The drawing under review shows one solid part. Ordinate dimensions are in mm from its lowest x, y, z. Round coordinates to 2 decimals unless told otherwise and drop trailing zeros. Write each loop counter-clockwise with the first axis right and the second up, starting at its lowest first coordinate (ties: lowest second). Pieces come first, ordered by that corner, then holes. Notation, with made-up numbers: M -6,52 L 46,52 A32 ccw 46,84 Z; hole C -6,2 d8. An arc over 180 degrees is marked long. One line per item, written item: value. Start each with the question number.
1) Take a section at C-C, the plane y = 4.5. Write out the cut boundary in (x, z) (3 decimals).
2) Wall thickness on probe 1 along X at (y, z) = (3, 62.5) (3 decimals); probe 2 along Z at (x, y) = (109.5, 2) (3 decimals); probe 3 along Z at (x, y) = (108.5, 6.25) (3 decimals): over which ranges is each line inside the solid? List them lowest first.
3) For P1, Ø4, axis at x = 117.475, z = 122.809, coming from the +Y side (3 decimals); P2, Ø3, axis at x = 3.175, z = 13.589, coming from the -Y side, all flat-tipped, find the tip position at first contact; note any pin that passes through.
4) Take a section at B-B, the plane z = 67. Write out the cut boundary in (x, y) (3 decimals).
5) Take a section at A-A, the plane x = 191. Write out the cut boundary in (y, z) (3 decimals), and give its area (3 significant figures).
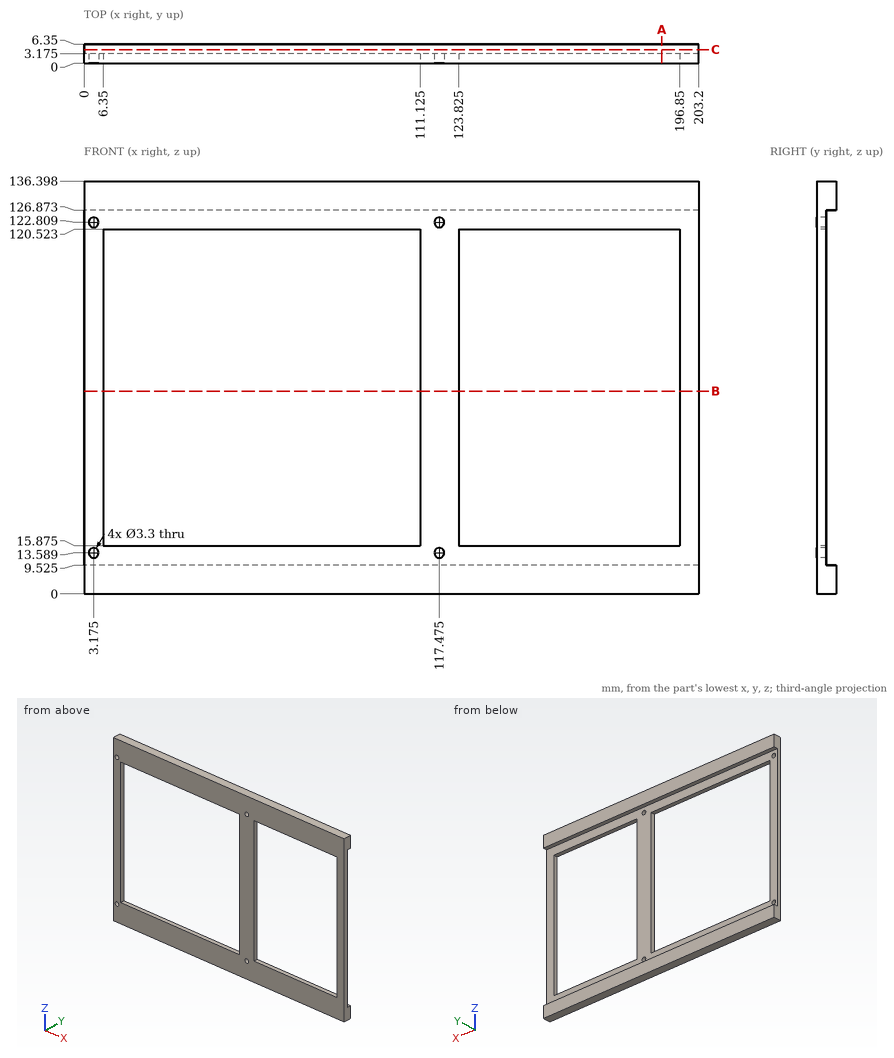
Checked values:
1. outline: M 0,0 L 203.2,0 L 203.2,9.525 L 0,9.525 Z; M 0,126.873 L 203.2,126.873 L 203.2,136.398 L 0,136.398 Z
2. probe 1: x = 0 to 6.35, 111.125 to 123.825, 196.85 to 203.2
2. probe 2: z = 0 to 15.875, 120.523 to 136.398
2. probe 3: z = 0 to 9.525, 126.873 to 136.398
3. P1: stops at y = 3.175
3. P2: passes through
4. outline: M 0,0 L 6.35,0 L 6.35,3.175 L 0,3.175 Z; M 111.125,0 L 123.825,0 L 123.825,3.175 L 111.125,3.175 Z; M 196.85,0 L 203.2,0 L 203.2,3.175 L 196.85,3.175 Z
5. outline: M 0,0 L 6.35,0 L 6.35,9.525 L 3.175,9.525 L 3.175,15.875 L 0,15.875 Z; M 0,120.523 L 3.175,120.523 L 3.175,126.873 L 6.35,126.873 L 6.35,136.398 L 0,136.398 Z
5. area: 161 mm2
